Can you work these out from the model? Positions are in its coordinate system, mm. A direction names the side the tool comes from. Coordinates: 2 decimals unless noted, no trailing zeros. Order: outer loops, then holes, each group sorted by start corner. A loop starts at its lowest first (then second) coordinate and runs counter-clockwise, first axis right, second up. Notation, with made-up numbers: (-1.5, 41) -> (38.5, 41) arc R31 ccw to (38.5, 71) -> close; hole circle Ø2 at (87.25, 52). An arc over 180 degrees is marked (long way). Return JSON: item names as keys, results as strings. Group by question number.
1) For pin 1 (3 mm diameter, centred on y = -2.5, z = 2.5, fed in from +X); pin 2 (4 mm diameter, centred on x = 0, y = 0, fed in from +Z); pin 3 (1 mm diameter, centred on y = 6, z = 5, fed in from +X), each with a flat end and sliding along its axis, tell me the tip position at first contact or that it passes through.
2) Thinking about a two-plate mould opening in X: for faces 4 (the cylindrical face through (-1.009, -7.684, 2.958)), 5 (the flat face through (4, 0, 0)), 6 (the cylindrical face through (2.954, -4.412, 3.042)), which applies, +X half, -X half, draft (parallel to the pull), parting line (faces both ways), or undercut?
3) If we section it at C-C, the plane x = -2.75: Please give me the cut outline in (y, z).
4) If we section it at B-B, the plane y = 0: Please give me the cut outline in (x, z), then the cut area to 3 significant figures.
5) If I drill on probe 1 along Y at (x, z) = (4.25, 3.5); probe 2 along X at (y, z) = (3.25, 2.5); probe 3 along Y at (x, z) = (0, 4.6), over which ranges is the centre line in solid material (lowest first)? Write a range as from..to.
6) If we section it at D-D, the plane z = 3.25: Please give me the cut outline in (x, y), then the cut area to 3 significant figures.
7) If we section it at A-A, the plane y = 4.25: Please give me the cut outline in (x, z).
8) For faces 1 (the flat face through (4, 0, 6)), 2 (the flat face through (-0.8, 2.794, 1.6)), 3 (the cylindrical face through (-0.33, 5.31, 1.57)), which set-ups out of +Z, -Z, +X, -X, +Y, -Y let a thin tool reach every point of the face, with its end or its side?
Autodesk Inventor part; units mm, degrees
ref_plane "YZ Plane" through (0, 0, 0) normal (1, 0, 0) x (0, 1, 0)
ref_plane "XZ Plane" through (0, 0, 0) normal (0, 1, 0) x (-1, 0, 0)
ref_plane "XY Plane" through (0, 0, 0) normal (0, 0, 1) x (1, 0, 0)
sketch "Sketch6" plane through (0, 0, 0) normal (0, 0, 1) x (1, 0, 0)
  circle A0 centre (0, 0) radius 7.75
  dimension "d44" = 15.5
extrude "Extrusion5" add sketch "Sketch6" along normal blind 6
sketch "Sketch7" plane through (0, 0, 0) normal (0, 0, -1) x (-1, 0, 0)
  point P0 (0, 0)
  point P1 (4.2426, 4.2426)
  point P2 (-4.2426, 4.2426)
  point P3 (-4.2426, -4.2426)
  point P4 (4.2426, -4.2426)
  dimension "d47" = 6
  dimension "d50" = 360
  dimension "d74" = 4.2426
hole "Hole4" at (-4.2426, 4.2426, 0) at (4.2426, 4.2426, 0) at (4.2426, -4.2426, 0) at (-4.2426, -4.2426, 0) direction (0, 0, 1) diameter 2.6 end through all
hole "Hole5" at (0, 0, 0) direction (0, 0, 1) diameter 6.731 end through all
sketch "Sketch8" plane through (0, 0, 0) normal (0, 0, -1) x (-1, 0, 0)
  circle A0 centre (0, 0) radius 3.3655
  line L0 (-1.8762, 2.794) -> (1.8762, 2.794)
  line L1 (1.8762, 2.794) -> (1.8762, 3.429)
  line L2 (1.8762, 3.429) -> (-1.8762, 3.429)
  line L3 (-1.8762, 3.429) -> (-1.8762, 2.794)
  dimension "d70" = 2.794
  dimension "d71" = 0.635
extrude "Extrusion6" add sketch "Sketch8" against normal blind 6 contours L0 A0 picked at (-0.1324, 2.9767)
sketch "Sketch9" plane through (-1.8762, 2.794, 0) normal (0, -1, 0) x (1, 0, 0)
  line L0 (0, 0) -> (0, 6)
  line L1 (3.7524, 0) -> (0, 0)
  point P0 (2, 3)
  dimension "d75" = 2
  dimension "d85" = 3
hole "Hole6" at (0.1238, 2.794, 3) direction (0, 1, 0) diameter 3 end through all
properties part number "omniWheelInsert"
Result sheet:
{
 "1": {"pin 1": "stops at x = 7.69", "pin 2": "passes through", "pin 3": "stops at x = 5.46"},
 "2": {"face 4": "parting line", "face 5": "draft", "face 6": "undercut"},
 "3": {"outline": "(-7.25, 0) -> (-1.94, 0) -> (-1.94, 6) -> (-7.25, 6) -> close; (1.94, 0) -> (7.25, 0) -> (7.25, 6) -> (1.94, 6) -> close"},
 "4": {"outline": "(-7.75, 0) -> (-3.37, 0) -> (-3.37, 6) -> (-7.75, 6) -> close; (3.37, 0) -> (7.75, 0) -> (7.75, 6) -> (3.37, 6) -> close", "area": "52.6 mm2"},
 "5": {"probe 1": "y = -6.48..-5.54, -2.94..2.94, 5.54..6.48", "probe 2": "x = -7.04..-5.08, -3.4..-1.29, 1.54..3.4, 5.08..7.04", "probe 3": "y = -7.75..-3.37, 2.79..7.75"},
 "6": {"outline": "(-1.88, 2.79) -> (-1.36, 2.79) -> (-1.36, 7.63) arc R7.75 ccw (long way) to (1.6, 7.58) -> (1.6, 2.79) -> (1.88, 2.79) arc R3.37 cw (long way) to start; hole circle Ø2.6 at (-4.24, -4.24); hole circle Ø2.6 at (-4.24, 4.24); hole circle Ø2.6 at (4.24, -4.24); hole circle Ø2.6 at (4.24, 4.24)", "area": "119 mm2"},
 "7": {"outline": "(-6.48, 0) -> (-5.54, 0) -> (-5.54, 6) -> (-6.48, 6) -> close; (-2.94, 0) -> (2.94, 0) -> (2.94, 6) -> (-2.94, 6) -> close; (5.54, 0) -> (6.48, 0) -> (6.48, 6) -> (5.54, 6) -> close; hole circle Ø3 at (0.12, 3)"},
 "8": {"face 1": "+Z, +X, -X, +Y, -Y", "face 2": "+Z, -Z", "face 3": "+Y"}
}
